Autodesk Inventor part; units mm, degrees
ref_plane "Work Plane1" through (17.4207, 0, 0) normal (0, 0, -1) x (-1, 0, 0)
ref_plane "YZ Plane" through (0, 0, 0) normal (1, 0, 0) x (0, 1, 0)
ref_plane "XZ Plane" through (0, 0, 0) normal (0, 1, 0) x (-1, 0, 0)
sketch "Sketch1" plane through (0, 0, 0) normal (0, 0, 1) x (1, 0, 0)
  line L0 (-1.2302, 0) -> (6.0384, 0)
  line L1 (2.6743, 4) -> (1.866, 5.4)
  line L2 (2.6743, 4) -> (5, 4) construction
  line L3 (5, 4) -> (5, 0) construction
  arc A0 (1.866, 5.4) -> (0, 4.9) centre (1, 4.9) ccw
  line L4 (2.6743, 4) -> (2.6743, 0)
  line L5 (0, -1.2232) -> (0, 7.3391)
  point P0 (0, 0)
  dimension "d2" = 8
  dimension "d4" = 11.8
  dimension "d5" = 1
  dimension "d15" = 5
  dimension "d16" = 30
revolve "Ring" add sketch "Sketch1" angle 360 about axis through (-10, 0, 0) along (1, 0, 0)
sketch "Sketch2" plane through (0, 0, 0) normal (-1, 0, 0) x (0, 0, 1)
  circle A0 centre (0, 0) radius 4.9
  line L0 (-4, -2.3094) -> (-4, 2.3094)
  line L1 (-4, 2.3094) -> (0, 4.6188)
  line L2 (0, 4.6188) -> (4, 2.3094)
  line L3 (4, 2.3094) -> (4, -2.3094)
  line L4 (4, -2.3094) -> (0, -4.6188)
  line L5 (0, -4.6188) -> (-4, -2.3094)
  circle A1 centre (0, 0) radius 4.9
  dimension "d6" = 9.2376
extrude "Body" add sketch "Sketch2" against normal blind 5 contours L0 L1 L2 L3 L4 L5
sketch "Sketch3" plane through (0, 0, 0) normal (0, 0, 1) x (1, 0, 0)
  line L0 (2.3171, 4.6188) -> (5, 4.6188)
  line L1 (5, 2.3094) -> (5, 4.6188)
  line L2 (0, -4.9) -> (0, 4.9)
  line L3 (-1, 0) -> (6, 0)
  line L4 (4.6427, 4.6188) -> (5, 4)
  dimension "d10" = 30
  dimension "d11" = 8
revolve "Chamfer1" cut sketch "Sketch3" angle 360 about axis through (-10, 0, 0) along (1, 0, 0)
sketch "Sketch4" plane through (0, 0, 0) normal (-1, 0, 0) x (0, 0, 1)
  circle A0 centre (0, 0) radius 4.9
hole "Thread" at (0, 0, 0) direction (1, 0, 0) diameter 4.134 end through all
chamfer "Chamfer2" distance 0.433 angle 30 1 edges at (0, 0, -2.067) measured on face at (0, 3.9032, -0.4739)
ref_plane "Work Plane1" through (17.4207, 0, 0) normal (0, 0, -1) x (-1, 0, 0)
chamfer "Chamfer3" distance 0.433 angle 45 1 edges at (5, 0, -2.067)
equation "\"d6\" = 1.1547 * SW"
equation "\"d7\" = KOH"
equation "\"d12\" = -0.5 * GD1 + 0.5 * NND"
equation "\"d46\" = -0.5 * GD1 + 0.5 * NND"
equation "\"d51\" = -0.5 * GD1 + 0.5 * NND"
equation "\"d2\" = SW"
equation "\"d4\" = LADI"
equation "\"d5\" = PHH"
equation "\"d15\" = KOH"
equation "\"d16\" = KEWI"
equation "\"d10\" = ANG1"
equation "\"d11\" = SW0"
equation "\"ANG1\" = 30deg"
equation "\"KEWI\" = 30deg"
equation "\"NND\" = 5"
equation "\"LADI\" = 11.8"
equation "\"SW\" = 8"
equation "\"PHH\" = RR"
equation "\"KOH\" = 5"
equation "\"SW0\" = SW"
equation "\"d1\" = LADI"
equation "\"d3\" = PHH"
equation "\"GUL\" = 0.541266 * PTC"
equation "\"RR\" = 1"
equation "\"THREADDIA\" = 5"
equation "\"TOA\" = 30deg"
equation "\"PTC\" = 0.8"
equation "\"RR1\" = 0.3"
equation "\"GAL\" = 0.541266 * PTC"
equation "\"E0\" = 1.155 * SW"
properties part number "ANSI B18.2.4.4M - M5 x 0.8" material "Steel, Mild"
Geometry check sheet. Reference: the model listing, model coordinates, mm. A direction names the side the tool comes from. Coordinates: 2 decimals unless noted, no trailing zeros. Loops run counter-clockwise (first coordinate to the right, second up) from the corner with the lowest first, then second, coordinate; pieces in that order, holes last. Notation, with made-up numbers: (25.25, 66.25) - (77.25, 66.25) arc R20 cw to (77.25, 78.25) - close; hole circle Ø10 at (28, 89.25). An arc over 180 degrees is marked (long way). Use one line per item in the form item = value. Start each with the question number.
Item 1: Section check A-A, the plane x = 3.2. Enter the section's corners in (y, z).
Item 2: Section check B-B, the plane x = 2.05. Enter the section's corners in (y, z).
Item 3: Tool access check on faces 4 (the face through (5, 2, 2)), 5 (the face through (3.64, -3.448, 2.028)), 6 (the face through (3.64, -3.48, -1.97)), 7 (the face through (2.534, -0.92, 4.142)), 8 (the face through (3.64, 3.448, -2.028)). Record the directions out of +Z, -Z, +X, -X, +Y, -Y that give a thin tool (end or side, any length) a straight path to the whole face; none if there is none.
Item 4: Section check C-C, the plane x = 0.7. Enter the section's corners in (y, z).
Item 5: Gauge pin test, flat ends, axial feed: pin 1 (1.3 mm diameter, centred on x = 4, y = 0.5, fed in from +Z); pin 2 (0.8 mm diameter, centred on x = 4.5, y = -0.5, fed in from -Z); pin 3 (1.5 mm diameter, centred on x = 4, z = 2, fed in from -Y). Record the tip position at first contact, or that the pin passes through.
Item 6: Mould release check, pull along Z, two halves, no side actions. Record for faces 1 (the face through (2.44, 1.26, -1.64)), 2 (the face through (4.913, 4.15, 0.01)), 3 (the face through (3.64, 3.48, 1.97)): +Z half, -Z half, draft (parallel to the pull), parting line (faces both ways), or undercut.
Item 7: Thickness scan on probe 1 along Z at (x, y) = (3.4, 0); probe 2 along Y at (x, z) = (0.5, -1.75); probe 3 along Z at (x, y) = (4.45, 1). Record the ranges inside material, lowest first.
Computed:
q1.outline = (-4.62, 0) - (-2.31, -4) - (2.31, -4) - (4.62, 0) - (2.31, 4) - (-2.31, 4) - close; hole circle Ø4.13 at (0, 0)
q2.outline = circle Ø10.16 at (0, 0); hole circle Ø4.13 at (0, 0)
q3.face_4 = +Z, -Z, +X, +Y, -Y
q3.face_5 = +Z, +X, -Y
q3.face_6 = -Z, +X, -Y
q3.face_7 = +X
q3.face_8 = -Z, +X, +Y
q4.outline = circle Ø11.71 at (0, 0); hole circle Ø4.13 at (0, 0)
q5.pin_1 = 4
q5.pin_2 = -4
q5.pin_3 = -3.9
q6.face_1 = undercut
q6.face_2 = parting line
q6.face_3 = +Z half
q7.probe_1 = -4 to -2.07, 2.07 to 4
q7.probe_2 = -5.49 to -1.1, 1.1 to 5.49
q7.probe_3 = -4 to -1.81, 1.81 to 4
